The listing builds one solid part. Answer for the finished solid, in the listing's coordinates (mm). A direction names the side the tool comes from. Coordinates: 2 decimals unless noted, no trailing zeros. Loops run counter-clockwise (first coordinate to the right, second up) from the corner with the lowest first, then second, coordinate; pieces in that order, holes last. Notation, with made-up numbers: (-29.75, -32) - (11.25, -32) arc R31 ccw to (11.25, 1) - close; hole circle Ø2 at (71, 80.5). An arc over 180 degrees is marked (long way). Put each result on its own line as item: value.
Autodesk Inventor part; units mm, degrees
ref_plane "YZ Plane" through (0, 0, 0) normal (1, 0, 0) x (0, 1, 0)
ref_plane "XZ Plane" through (0, 0, 0) normal (0, 1, 0) x (-1, 0, 0)
ref_plane "XY Plane" through (0, 0, 0) normal (0, 0, 1) x (1, 0, 0)
sketch "Sketch1" plane through (0, 0, 0) normal (0, 0, 1) x (1, 0, 0)
  line L0 (-125.5, -166.9563) -> (125.5, -166.9563)
  line L1 (125.5, -166.9563) -> (125.5, 166.9563)
  line L2 (125.5, 166.9563) -> (-125.5, 166.9563)
  line L3 (-125.5, 166.9563) -> (-125.5, -166.9563)
  line L4 (-125.5, -166.9563) -> (125.5, 166.9563) construction
  line L5 (125.5, -166.9563) -> (-125.5, 166.9563) construction
  point P0 (0, 0)
  dimension "d0" = 251
  dimension "d1" = 333.9125
extrude "Extrusion1" add sketch "Sketch1" along normal blind 3.15
sketch "Sketch2" plane through (0, 0, 0) normal (0, 0, -1) x (-1, 0, 0)
  line L0 (125.5, -166.9563) -> (-125.5, -166.9563)
  line L1 (-125.5, 166.9563) -> (-122.35, 166.9563)
  line L2 (-122.35, 166.9563) -> (-122.35, -166.9563)
  line L3 (-122.35, -166.9563) -> (-125.5, -166.9563)
  line L4 (-125.5, -166.9563) -> (-125.5, 166.9563)
  line L5 (125.5, 166.9563) -> (122.35, 166.9563)
  line L6 (122.35, 166.9563) -> (122.35, -166.9563)
  line L7 (122.35, -166.9563) -> (125.5, -166.9563)
  line L8 (125.5, -166.9563) -> (125.5, 166.9563)
  line L9 (-122.35, 166.9563) -> (122.35, 166.9563)
  line L10 (122.35, 166.9563) -> (122.35, 163.8062)
  line L11 (122.35, 163.8062) -> (-122.35, 163.8062)
  line L12 (-122.35, 163.8062) -> (-122.35, 166.9563)
  point P0 (0, 0)
  dimension "d4" = 3.15
  dimension "d5" = 3.15
  dimension "d6" = 3.15
extrude "Extrusion2" add sketch "Sketch2" along normal blind 88.65 contours L0 L6 L5 L8 | L0 L4 L1 L2 | L11 L2 L9 L6
equation "\"d0\" = door_x"
equation "\"d1\" = door_z"
equation "\"d2\" = clear_acrylic"
equation "\"d4\" = clear_acrylic"
equation "\"d5\" = clear_acrylic"
equation "\"d6\" = clear_acrylic"
equation "\"d7\" = window_y"
equation "\"sm_thickness\" = 1.5875"
equation "\"al_thickness\" = 1.5875"
equation "\"bend_factor\" = 2.26205"
equation "\"al_bend\" = 3.591"
equation "\"sm_bend\" = 3.591"
equation "\"very_thick_acrylic\" = 9.45"
equation "\"thick_acrylic\" = 5.88"
equation "\"thin_acrylic\" = 3.15"
equation "\"clear_acrylic\" = 3.15"
equation "\"wood_thickness\" = 6.72"
equation "\"m3_diameter\" = 3"
equation "\"m3_head\" = 6"
equation "\"m4_diameter\" = 4"
equation "\"m5_diameter\" = 5"
equation "\"m5_head\" = 10.3"
equation "\"rivet_diameter\" = 3.3"
equation "\"brass_insert_drill\" = 4"
equation "\"m5_brass_insert_drill\" = 6.7"
equation "\"m3_press_nut_drill\" = 4.5"
equation "\"m5_press_nut_drill\" = 6.5"
equation "\"laser_body_diameter\" = 12"
equation "\"carrier_y\" = 251"
equation "\"carrier_y2\" = 76.825"
equation "\"carrier_z\" = 12"
equation "\"carrier_z2\" = 25"
equation "\"visor_x\" = 257.3"
equation "\"visor_y\" = 108.65"
equation "\"window_z\" = 333.9125"
equation "\"window_y\" = 88.65"
equation "\"window_overlap\" = 48"
equation "\"acrylic_into_frame\" = 5"
equation "\"door_x\" = 251"
equation "\"door_z\" = 333.9125"
equation "\"door_overlap\" = 48"
equation "\"reservoir_x\" = 201"
equation "\"reservoir_y\" = 201"
equation "\"linear_bearing_spacing\" = 271"
equation "\"tray_border\" = 25"
equation "\"tray_x\" = 251"
equation "\"tray_y\" = 251"
equation "\"bed_z\" = 25"
equation "\"crane_z2\" = 12"
equation "\"switch_spacing\" = 19"
equation "\"frame_top_z\" = 385"
equation "\"frame_bottom_z\" = 275"
equation "\"frame_total_z\" = 661.5875"
equation "\"frame_x\" = 350.2"
equation "\"frame_face_y\" = 45"
equation "\"frame_border\" = 46.35"
equation "\"frame_foot_z\" = 12"
equation "\"frame_screw_from_center\" = 25"
equation "\"laser_y_offset\" = 19.4"
equation "\"laser_diameter\" = 12"
equation "\"laser_z_offset\" = 55"
equation "\"laser_y\" = 15"
equation "\"laser_z\" = 75"
equation "\"laser_gap\" = 1"
equation "\"subframe_x\" = 66"
equation "\"subframe_y\" = 55"
equation "\"galvo_frame_x\" = 66"
equation "\"galvo_frame_z\" = 65"
equation "\"galvo_frame_y_offset\" = 27.5"
equation "\"drawer_x\" = 257.3"
equation "\"drawer_y\" = 85.2375"
equation "\"drawer_z\" = 278.175"
equation "\"drawer_support_from_top\" = 48"
equation "\"drawer_screw_z\" = 145"
equation "\"drawer_screw_from_center\" = 55"
equation "\"nema17_x\" = 43"
properties part number "window2"
1) The part is cut by section A-A (z = -34). Give the vertices of the cut face in (x, y).
Found:
outline: (-125.5, -166.96) - (-122.35, -166.96) - (-122.35, 163.81) - (122.35, 163.81) - (122.35, -166.96) - (125.5, -166.96) - (125.5, 166.96) - (-125.5, 166.96) - close
2) Each of these flat-tipped pins is pushed along its axis until it touches: pin 1 (12 mm diameter, centred on x = 73, y = -33.5, fed in from -Z); pin 2 (6 mm diameter, centred on x = 11.5, z = -31, fed in from -Y). Where does it stop, or does it pass through?
Found:
pin 1: stops at z = 0
pin 2: stops at y = 163.81
3) The part is cut by section C-C (x = 71.5). Give the vertices of the cut face in (y, z).
Found:
outline: (-166.96, 0) - (163.81, 0) - (163.81, -88.65) - (166.96, -88.65) - (166.96, 3.15) - (-166.96, 3.15) - close
4) For a pull along X with two mould halves and no side action, classify faces 3 (the face through (125.5, -2, -43)), 4 (the face through (-1, -166.956, 1)), 5 (the face through (-2, 163.806, -44)), 6 (the face through (-2, 1, 0)) as pulls with the +X half, pulls with the -X half, needs draft (parallel to the pull), parting line crosses it, or undercut.
Found:
face 3: pulls with the +X half
face 4: needs draft
face 5: undercut
face 6: undercut
5) Straight lines are drawn through the part: L1, parallel to X at y = 26, z = -42.5; L2, parallel to Y at x = 107.5, z = -48; L3, parallel to Z at x = -66, y = 129.5. For each, find the intervals that lie inside material, in ascending order. Write a range as [from, to].
Found:
L1: x = [-125.5, -122.35], [122.35, 125.5]
L2: y = [163.81, 166.96]
L3: z = [0, 3.15]
6) For faces 1 (the face through (2, 166.956, -43)), 2 (the face through (-122.35, 1, -44)), determine the directions among +Z, -Z, +X, -X, +Y, -Y from which every point of the face is accessible in a straight line to the end or side of a thin tool.
Found:
face 1: +Z, -Z, +X, -X, +Y
face 2: -Z, -Y
7) The part is cut by section B-B (y = -61). Give the vertices of the cut face in (x, z), and give its area (3 significant figures).
Found:
outline: (-125.5, -88.65) - (-122.35, -88.65) - (-122.35, 0) - (122.35, 0) - (122.35, -88.65) - (125.5, -88.65) - (125.5, 3.15) - (-125.5, 3.15) - close
area: 1,350 mm^2
